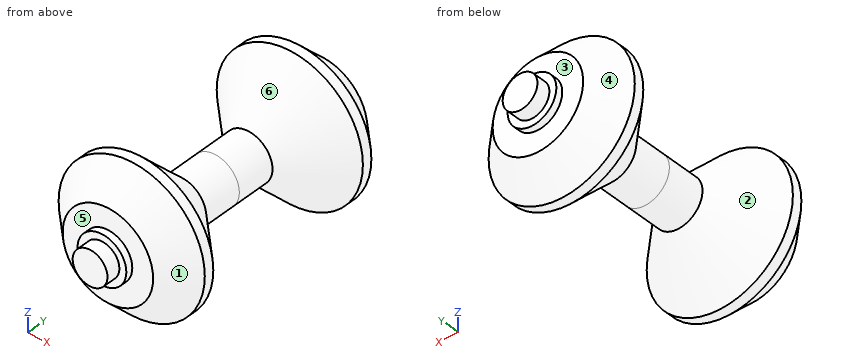
```python
from build123d import *


with BuildPart() as part:
    # Sketch1 → Revolve1 (revolve)
    with BuildSketch(Plane.XY):
        Polygon((0, 21), (0, 0), (3.5, 0), (3.5, 5.571782079), (10.5, 12.571782079), (10.5, 14), (6.5, 18), (3.5, 18), (3.5, 19), (2.5, 19), (2.5, 21), align=None)
    revolve1 = revolve(axis=Axis((0, 21, 0), (0, -1, 0)))

    # Mirror1: Revolve1 across plane
    add(revolve1.mirror(Plane.ZX))


solid = part.part
```
Here's how the part is built. I have some questions about the finished solid (model axes, mm). Face numbers are marked on the shaded views. A direction names the side the tool comes from. Round coordinates to 2 decimals unless told otherwise and drop trailing zeros. Order: outer loops, then holes, each group sorted by start corner. A loop starts at its lowest first (then second) coordinate and runs counter-clockwise, first axis right, second up. Notation, with made-up numbers: M -30,62.25 L 19,62.25 A26 ccw 19,84.25 Z; hole C -38,82.25 d3. An arc over 180 degrees is marked long. Answer in a Markdown table with one row per item.
Item 1: For the marked faces 1, 2 and 3, which set-ups out of +Z, -Z, +X, -X, +Y, -Y let a thin tool reach every point of the face, with its end or its side?
A:
| item | result |
|---|---|
| face 1 | -Y |
| face 2 | none |
| face 3 | +Y |
Item 2: Imagine slicing it at D-D, the plane y = -1. Write out the boundary of the cut face in (x, z), and give its area (3 significant figures).
A:
| item | result |
|---|---|
| outline | C 0,0 d7 |
| area | 38.5 mm2 |
Item 3: If I drill on L1, parallel to Y at x = -0.75, z = -8.5; L2, parallel to Y at x = -5.75, z = -4; L3, parallel to X at y = 13.5, z = 9.5, over which ranges is the centre line in solid material (lowest first)? Write a range as from..to.
A:
| item | result |
|---|---|
| L1 | y = -15.97..-10.6, 10.6..15.97 |
| L2 | y = -17.5..-9.08, 9.08..17.5 |
| L3 | x = -4.47..4.47 |
Item 4: I'm going to push flat-ended pins straight in: pin 1 (5 mm diameter, centred on y = -1, z = -7.5, fed in from +X); pin 2 (3 mm diameter, centred on y = 6.5, z = -1.5, fed in from +X); pin 3 (1.5 mm diameter, centred on x = 5.5, z = -6, fed in from +Y); pin 4 (8 mm diameter, centred on x = 5.5, y = -14, fed in from -Z). Where does each tip first touch, or does it pass through?
A:
| item | result |
|---|---|
| pin 1 | passes through |
| pin 2 | stops at x = 5.77 |
| pin 3 | stops at y = 17.11 |
| pin 4 | stops at z = -10.39 |
Item 5: Thinking about a two-plate mould opening in Y: for the marked faces 4, 5 and 6, which applies, +Y half, -Y half, draft (parallel to the pull), parting line (faces both ways), or undercut?
A:
| item | result |
|---|---|
| face 4 | +Y half |
| face 5 | -Y half |
| face 6 | undercut |
Item 6: Imagine slicing it at C-C, the plane y = -16. Write out the boundary of the cut face in (x, z), and give its area (3 significant figures).
A:
| item | result |
|---|---|
| outline | C 0,0 d17 |
| area | 227 mm2 |
